```python
from build123d import *

# Parameters (mm, degrees)
IZIM1_R                              = 1.5
N_PANEL_DEPTH                        = 2
VIDA_DELIKLERI_45DERECE_PAH_1MM_SIZE = 1
IZIM2_W                              = 70.48450085
IZIM2_H                              = 120
EKRAN_VE_KONTROLC_DELIKLERI_DEPTH    = 2
FILLET1_R                            = 1


with BuildPart() as part:
    # Çizim1 → Ön Panel (new body)
    with BuildSketch(Plane(origin=(0, 0, 0), x_dir=(0, 1, 0), z_dir=(0, 0, 1))):
        with BuildLine():
            Line((-1, 0), (-183.6, 0))
            ThreePointArc((-183.6, 0), (-184.307106781, -0.292893219), (-184.6, -1))
            Line((-184.6, -1), (-184.6, -89))
            ThreePointArc((-184.6, -89), (-184.307106781, -89.707106781), (-183.6, -90))
            Line((-183.6, -90), (-1, -90))
            ThreePointArc((-1, -90), (-0.292893219, -89.707106781), (0, -89))
            Line((0, -89), (0, -1))
            ThreePointArc((0, -1), (-0.292893219, -0.292893219), (-1, 0))
        make_face()
        with Locations((-179.693599404, -4.906400596)):
            Circle(IZIM1_R, mode=Mode.SUBTRACT)
        with Locations((-4.906400596, -4.906400596)):
            Circle(IZIM1_R, mode=Mode.SUBTRACT)
        with Locations((-179.693599404, -85.093599404)):
            Circle(IZIM1_R, mode=Mode.SUBTRACT)
        with Locations((-4.906400596, -85.093599404)):
            Circle(IZIM1_R, mode=Mode.SUBTRACT)
    extrude(amount=N_PANEL_DEPTH)

    # Vida Delikleri 45derece Pah 1mm
    vida_delikleri_45derece_pah_1mm_edges = [part.edges().sort_by_distance(p)[0] for p in [
        (85.093599404, -6.406400596, 2),
        (4.906400596, -6.406400596, 2),
        (4.906400596, -181.193599404, 2),
        (85.093599404, -181.193599404, 2),
    ]]
    chamfer(vida_delikleri_45derece_pah_1mm_edges, length=VIDA_DELIKLERI_45DERECE_PAH_1MM_SIZE)

    # Çizim2 → Ekran ve Kontrolcü delikleri (cut)
    with BuildSketch(Plane.XY.offset(2)):
        with Locations((45, -69.798366298)):
            Rectangle(IZIM2_W, IZIM2_H)
        Polygon((40.317046277, -138.653704662), (40.317046277, -134.653704662), (3.616207615, -134.653704662), (3.616207615, -172.224363873), (80.242250425, -172.224363873), (80.242250425, -138.653704662), align=None)
    extrude(amount=-EKRAN_VE_KONTROLC_DELIKLERI_DEPTH, mode=Mode.SUBTRACT)

    # Fillet1
    fillet1_edges = [part.edges().sort_by_distance(p)[0] for p in [
        (0, -92.3, 2),
        (45, -184.6, 2),
        (90, -92.3, 2),
        (45, 0, 2),
    ]]
    fillet(fillet1_edges, radius=FILLET1_R)


solid = part.part
```
Check sheet for the modelled part. Datum: model origin and axes. Units: mm. Round coordinates to 2 decimals unless told otherwise and drop trailing zeros. Order: outer loops, then holes, each group sorted by start corner. A loop starts at its lowest first (then second) coordinate and runs counter-clockwise, first axis right, second up. Notation, with made-up numbers: M 24.5,83.5 L 76.5,83.5 A19 cw 76.5,92.5 Z; hole C -38.5,-6.75 d8. An arc over 180 degrees is marked long. Answer in a Markdown table with one row per item.
(1) Section check C-C on z = 0.5. Record the boundary of the cut face in (x, y), plus the area to 3 significant figures.
Findings:
| item | result |
|---|---|
| outline | M 0,-183.6 A1 ccw 1,-184.6 L 89,-184.6 A1 ccw 90,-183.6 L 90,-1 A1 ccw 89,0 L 1,0 A1 ccw 0,-1 Z; hole C 4.91,-179.69 d3; hole C 4.91,-4.91 d3; hole M 3.62,-172.22 L 80.24,-172.22 L 80.24,-138.65 L 40.32,-138.65 L 40.32,-134.65 L 3.62,-134.65 Z; hole M 9.76,-129.8 L 80.24,-129.8 L 80.24,-9.8 L 9.76,-9.8 Z; hole C 85.09,-179.69 d3; hole C 85.09,-4.91 d3 |
| area | 5,410 mm^2 |
(2) Section check B-B on x = 43. Record the boundary of the cut face in (y, z), plus the area to 3 significant figures.
Findings:
| item | result |
|---|---|
| outline | M -184.6,0 L -172.22,0 L -172.22,2 L -183.6,2 A1 ccw -184.6,1 Z; M -138.65,0 L -129.8,0 L -129.8,2 L -138.65,2 Z; M -9.8,0 L 0,0 L 0,1 A1 ccw -1,2 L -9.8,2 Z |
| area | 61.6 mm^2 |
(3) Section check D-D on x = 15. Record the boundary of the cut face in (y, z), plus the area to 3 significant figures.
Findings:
| item | result |
|---|---|
| outline | M -184.6,0 L -172.22,0 L -172.22,2 L -183.6,2 A1 ccw -184.6,1 Z; M -134.65,0 L -129.8,0 L -129.8,2 L -134.65,2 Z; M -9.8,0 L 0,0 L 0,1 A1 ccw -1,2 L -9.8,2 Z |
| area | 53.6 mm^2 |
(4) Section check A-A on y = -62. Record the boundary of the cut face in (x, z), plus the area to 3 significant figures.
Findings:
| item | result |
|---|---|
| outline | M 0,0 L 9.76,0 L 9.76,2 L 1,2 A1 ccw 0,1 Z; M 80.24,0 L 90,0 L 90,1 A1 ccw 89,2 L 80.24,2 Z |
| area | 38.6 mm^2 |
(5) Gauge pin test, flat end, axial feed: pin 1 (4 mm diameter, centred on x = 85.09, y = -179.69, fed in from -Z). Record the tip position at first contact, or that the pin passes through.
Findings:
| item | result |
|---|---|
| pin 1 | stops at z = 0 |
(6) Material ranges on line 1 along Y through (x, z) = (78.5, 1.1); line 2 along X through (y, z) = (-23, 0.2); line 3 along Y through (x, z) = (12, 1), recorded low to high. Write a range as from..to.
Findings:
| item | result |
|---|---|
| line 1 | y = -184.59..-172.22, -138.65..-129.8, -9.8..-0.01 |
| line 2 | x = 0..9.76, 80.24..90 |
| line 3 | y = -184.6..-172.22, -134.65..-129.8, -9.8..0 |
